Part model, mm, in its own coordinate system. Face numbers are marked on the shaded views. A direction names the side the tool comes from. Round coordinates to 2 decimals unless told otherwise and drop trailing zeros. Order: outer loops, then holes, each group sorted by start corner. A loop starts at its lowest first (then second) coordinate and runs counter-clockwise, first axis right, second up. Notation, with made-up numbers: (37.25, 89) -> (60.25, 89) arc R17 cw to (60.25, 101) -> close; hole circle Ø4 at (-3, -20). An arc over 180 degrees is marked (long way). Use CSV: the item, a comma, the result in double quotes.
Autodesk Inventor part; units mm, degrees
ref_plane "YZ Plane" through (0, 0, 0) normal (1, 0, 0) x (0, 1, 0)
ref_plane "XZ Plane" through (0, 0, 0) normal (0, 1, 0) x (-1, 0, 0)
ref_plane "XY Plane" through (0, 0, 0) normal (0, 0, 1) x (1, 0, 0)
sketch "Esquisse1" plane through (0, 0, 0) normal (0, 0, 1) x (1, 0, 0)
  line L0 (0, 0) -> (0, 25.5)
  line L1 (0, 25.5) -> (-12, 25.5)
  line L2 (-12, 25.5) -> (-18, 15.5)
  line L3 (-18, 15.5) -> (-18, 0)
  line L4 (-18, 0) -> (0, 0)
  dimension "d0" = 18
  dimension "d1" = 25.5
  dimension "d2" = 15.5
  dimension "d3" = 12
extrude "Extrusion1" add sketch "Esquisse1" along normal blind 10
sketch "Esquisse2" plane through (0, 0, 10) normal (0, 0, 1) x (1, 0, 0)
  circle A0 centre (-7.6, 15) radius 4.5
  line L0 (-18, 0) -> (0, 0)
  line L1 (0, 0) -> (0, 25.5)
  dimension "d6" = 9
  dimension "d7" = 15
  dimension "d8" = 7.6
extrude "Extrusion2" cut sketch "Esquisse2" against normal through all
sketch "Esquisse3" plane through (-18, 0, 0) normal (-1, 0, 0) x (0, 0, 1)
  circle A0 centre (5, 10.5) radius 1.5
  circle A1 centre (5, 3.5) radius 1.5
  line L0 (10, 15.5) -> (10, 0)
  line L1 (0, 15.5) -> (0, 0)
  line L2 (0, 0) -> (10, 0)
  dimension "d11" = 3
  dimension "d12" = 10
  dimension "d13" = 5
  dimension "d14" = 7
  dimension "d15" = 3.5
extrude "Extrusion3" cut sketch "Esquisse3" against normal blind 5
sketch "Esquisse4" plane through (-18, 0, 0) normal (0, -1, 0) x (1, 0, 0)
  circle A0 centre (8, 5) radius 1.5
  circle A1 centre (15, 5) radius 1.5
  line L0 (0, 10) -> (18, 10)
  line L1 (0, 0) -> (18, 0)
  line L2 (18, 0) -> (18, 10)
  dimension "d18" = 10
  dimension "d19" = 5
  dimension "d20" = 7
  dimension "d21" = 3
  dimension "d22" = 3
extrude "Extrusion4" cut sketch "Esquisse4" against normal blind 5
fillet "Congé1" radius 4 3 edges at (-12, 25.5, 5) (0, 25.5, 5) (-18, 15.5, 5)
equation "\"d13\" = 0.5 * d12"
equation "\"d19\" = 0.5 * d18"
properties part number "PilierCentral" material "Plastique ABS"
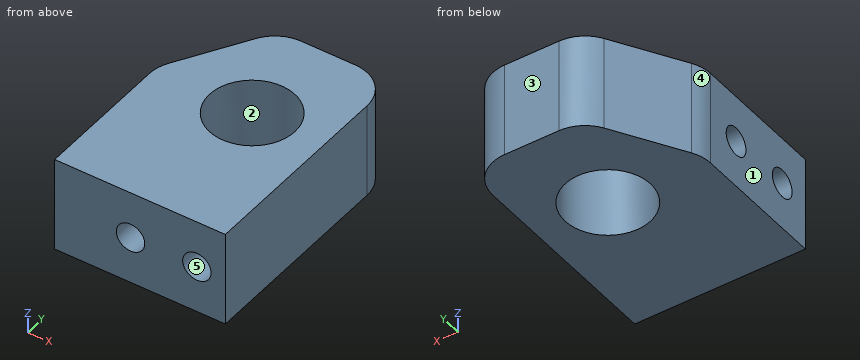
(1) Cut at A-A, the plane x = -7.6. Give the cut face in (y, z).
Reply:
outline,"(0, 0) -> (10.5, 0) -> (10.5, 10) -> (0, 10) -> close; (19.5, 0) -> (25.5, 0) -> (25.5, 10) -> (19.5, 10) -> close"
(2) Probe probe 1 along Z at (x, y) = (-3, 1.35); probe 2 along Y at (x, z) = (-14.05, 5); probe 3 along Y at (x, z) = (-5, 8.25). List the from-to ranges inside material, lowest first. Write a range as [from, to].
Reply:
probe 1,"[0, 3.5], [6.5, 10]"
probe 2,"[0, 2], [5, 9], [12, 22.08]"
probe 3,"[0, 11.33], [18.67, 25.5]"
(3) Drop a flat-ended pin along its axis: P1, Ø4, axis at x = -13, z = 5, coming from the +Y side. Give the stop position or say it passes through.
Reply:
P1,"y = 25.29"
(4) Cut at C-C, the plane y = 15. Give the cut face in (x, z).
Reply:
outline,"(-17.95, 0) -> (-12.1, 0) -> (-12.1, 10) -> (-17.95, 10) -> close; (-3.1, 0) -> (0, 0) -> (0, 10) -> (-3.1, 10) -> close"
(5) Pull direction X, two halves, no side cores. Call the marked faces 1, 2 and 3: released by +X, released by -X, zero draft, split by the parting line, or undercut.
Reply:
face 1,"released by -X"
face 2,"undercut"
face 3,"zero draft"
(6) Cut at B-B, the plane z = 5. Give the cut face in (x, y), then the cut area to 3 significant figures.
Reply:
outline,"(-18, 0) -> (-11.5, 0) -> (-11.5, 5) -> (-8.5, 5) -> (-8.5, 0) -> (-4.5, 0) -> (-4.5, 5) -> (-1.5, 5) -> (-1.5, 0) -> (0, 0) -> (0, 21.5) arc R4 ccw to (-4, 25.5) -> (-9.74, 25.5) arc R4 ccw to (-13.17, 23.56) -> (-17.43, 16.45) arc R4 ccw to (-18, 14.39) -> (-18, 12) -> (-13, 12) -> (-13, 9) -> (-18, 9) -> (-18, 5) -> (-13, 5) -> (-13, 2) -> (-18, 2) -> close; hole circle Ø9 at (-7.6, 15)"
area,"301 mm2"
(7) Which spindle directions (+Z, -Z, +X, -X, +Y, -Y) get a long thin tool onto all of the face, cutting with end or side? Do the marked faces 4 and 5. Say none if no direction does.
Reply:
face 4,"+Z, -Z, -X, +Y"
face 5,"-Y"
(8) Cut at D-D, the plane x = -15.25. Give the cut face in (y, z), then the cut area to 3 significant figures.
Reply:
outline,"(0, 0) -> (20.08, 0) -> (20.08, 10) -> (0, 10) -> close; hole circle Ø3 at (3.5, 5); hole circle Ø3 at (10.5, 5)"
area,"187 mm2"
